```python
from build123d import *

# Parameters (mm, degrees)
SKETCH1_W           = 20
SKETCH1_H           = 50
BOSS_EXTRUDE1_DEPTH = 1.2
SKETCH2_R           = 1.5
CUT_EXTRUDE1_DEPTH  = 2.2
SKETCH3_W           = 2.5
SKETCH3_H           = 10
SKETCH3_W_2         = 2.05
SKETCH3_H_2         = 3.15
SKETCH3_W_3         = 2.1
SKETCH3_H_3         = 4.1
SKETCH3_W_4         = 4.1
SKETCH3_H_4         = 2.05
SKETCH3_W_5         = 3
SKETCH3_H_5         = 1.1
SKETCH3_W_6         = 4
SKETCH3_H_6         = 4
SKETCH3_W_7         = 1.75
SKETCH3_H_7         = 3.5
BOSS_EXTRUDE2_DEPTH = 1.5


with BuildPart() as part:
    # Sketch1 → Boss-Extrude1 (new body)
    with BuildSketch(Plane(origin=(0, 0, 0), x_dir=(1, 0, 0), z_dir=(0, 1, 0))):
        Rectangle(SKETCH1_W, SKETCH1_H)
    extrude(amount=BOSS_EXTRUDE1_DEPTH)

    # Sketch2 → Cut-Extrude1 (cut, through all)
    with BuildSketch(Plane.XZ):
        with Locations((0, 17.5)):
            Circle(SKETCH2_R)
        with Locations((0, -17.5)):
            Circle(SKETCH2_R)
    extrude(amount=-CUT_EXTRUDE1_DEPTH, mode=Mode.SUBTRACT)

    # Sketch3 → Boss-Extrude2 (add)
    with BuildSketch(Plane.XZ):
        with Locations((5.75, -16.5)):
            Rectangle(SKETCH3_W, SKETCH3_H)
        with Locations((-5.975, -13.225)):
            Rectangle(SKETCH3_W_2, SKETCH3_H_2)
        with Locations((-4.95, -1.1)):
            Rectangle(SKETCH3_W_3, SKETCH3_H_3)
        with Locations((0.05, -2.425)):
            Rectangle(SKETCH3_W_4, SKETCH3_H_4)
        with Locations((0, 2.5)):
            Rectangle(SKETCH3_W_5, SKETCH3_H_5)
        with Locations((8, 0)):
            Rectangle(SKETCH3_W_6, SKETCH3_H_6)
        with Locations((-6.675, 9.35)):
            Rectangle(SKETCH3_W_7, SKETCH3_H_7)
    extrude(amount=-BOSS_EXTRUDE2_DEPTH)


solid = part.part
```
The model under review builds one solid part; all positions refer to its coordinate system, in mm. Coordinates: 2 decimals unless noted, no trailing zeros. Write each loop counter-clockwise with the first axis right and the second up, starting at its lowest first coordinate (ties: lowest second). Pieces come first, ordered by that corner, then holes. Notation, with made-up numbers: (-32.75, 6) -> (4.25, 6) arc R24 cw to (4.25, 29) -> close; hole circle Ø4 at (46.5, -6.5). An arc over 180 degrees is marked (long way). One line per item, written item: value. Start each with the question number.
Q1. To check wall thickness, follow probe 1 along Z at (x, y) = (0, 0.85); probe 2 along Y at (x, z) = (-5.75, 16). State the ranges of each line that lie inside material, in increasing order.
Q2. Add section D-D, the plane x = 5.5. Give the boundary of the cut face in (y, z), then the cut area to 3 significant figures.
Q3. Clearance check with a flat-ended pin moving along its axis: P1, Ø3, axis at x = 7, z = 10.5, coming from the +Y side. State where the tip first meets the part, or that it passes through.
Q4. Add section A-A, the plane z = -17.5. Give the boundary of the cut face in (x, y), then the cut area to 4 significant figures.
Q5. The part is to be moulded in two halves that separate along Z. For faces 1 (the face through (0, 1, 19)), 2 (the face through (0, 1, -25)), 3 (the face through (-6, 1.5, -13)), 4 (the face through (0, 1, 25)), say which applies: +Z half, -Z half, draft (parallel to the pull), parting line (faces both ways), or undercut.
Q6. Add section C-C, the plane z = 17.5. Give the boundary of the cut face in (x, y), then the cut area to 3 significant figures.
Q7. Add section B-B, the plane x = 0. Give the boundary of the cut face in (y, z).
Response:
1. probe 1: -25 to -19, -16 to 16, 19 to 25
1. probe 2: 0 to 1.2
2. outline: (0, -25) -> (1.2, -25) -> (1.2, -21.5) -> (1.5, -21.5) -> (1.5, -11.5) -> (1.2, -11.5) -> (1.2, 25) -> (0, 25) -> close
2. area: 63.0 mm²
3. P1: y = 1.2
4. outline: (-10, 0) -> (-1.5, 0) -> (-1.5, 1.2) -> (-10, 1.2) -> close; (1.5, 0) -> (10, 0) -> (10, 1.2) -> (7, 1.2) -> (7, 1.5) -> (4.5, 1.5) -> (4.5, 1.2) -> (1.5, 1.2) -> close
4. area: 21.15 mm²
5. face 1: undercut
5. face 2: -Z half
5. face 3: draft
5. face 4: +Z half
6. outline: (-10, 0) -> (-1.5, 0) -> (-1.5, 1.2) -> (-10, 1.2) -> close; (1.5, 0) -> (10, 0) -> (10, 1.2) -> (1.5, 1.2) -> close
6. area: 20.4 mm²
7. outline: (0, -25) -> (1.2, -25) -> (1.2, -19) -> (0, -19) -> close; (0, -16) -> (1.2, -16) -> (1.2, -3.45) -> (1.5, -3.45) -> (1.5, -1.4) -> (1.2, -1.4) -> (1.2, 1.95) -> (1.5, 1.95) -> (1.5, 3.05) -> (1.2, 3.05) -> (1.2, 16) -> (0, 16) -> close; (0, 19) -> (1.2, 19) -> (1.2, 25) -> (0, 25) -> close
